Autodesk Inventor part; units mm, degrees
ref_plane "YZ Plane" through (0, 0, 0) normal (1, 0, 0) x (0, 1, 0)
ref_plane "XZ Plane" through (0, 0, 0) normal (0, 1, 0) x (-1, 0, 0)
ref_plane "XY Plane" through (0, 0, 0) normal (0, 0, 1) x (1, 0, 0)
sketch "Sketch1" plane through (0, 0, 0) normal (0, 0, 1) x (1, 0, 0)
  arc A0 (1.4, -1.4283) -> (-1.4, -1.4283) centre (0, 0) ccw
  line L0 (-1.4, -1.4283) -> (-1.4, -10)
  line L1 (-1.4, -10) -> (1.4, -10)
  line L2 (1.4, -10) -> (1.4, -1.4283)
  point P0 (0, -10)
  dimension "d0" = 4
  dimension "d1" = 2.8
  dimension "d2" = 12
extrude "Extrusion1" add sketch "Sketch1" along normal blind 0.3
fillet "Fillet1" radius 1.4 2 edges at (1.4, -10, 0.15) (-1.4, -10, 0.15)
sketch "Sketch2" plane through (0, 0, 0.3) normal (0, 0, 1) x (1, 0, 0)
  circle A0 centre (0, -3.9283) radius 0.9
  point P0 (1.4, -1.4283)
  dimension "d6" = 1.8
  dimension "d7" = 2.5
extrude "Extrusion2" cut sketch "Sketch2" against normal through all
properties material "Brass, Soft Yellow"
Geometry: final body of the model. Coordinates: model frame, mm. Round coordinates to 2 decimals unless told otherwise and drop trailing zeros. Order: outer loops, then holes, each group sorted by start corner. A loop starts at its lowest first (then second) coordinate and runs counter-clockwise, first axis right, second up. Notation, with made-up numbers: (-17.75, -32) -> (-0.75, -32) arc R34 cw to (-0.75, 7) -> close; hole circle Ø9 at (-13.75, -0.5). An arc over 180 degrees is marked (long way). Put each result on its own line as item: value. Start each with the question number.
Q1. Section D-D on y = -8.75. Return the cut outline in (x, z), and give its area (3 significant figures).
Q2. First-contact query: pin 1 (1 mm diameter, centred on x = 1.5, y = -3, fed in from -Z). Flat tip, straight axial feed; report the tip coordinate or a pass-through.
Q3. Section A-A on y = -3.5. Return the cut outline in (x, z), and give its area (3 significant figures).
Q4. Line query: probe 1 along X at (y, z) = (-6.5, 0.15); probe 2 along Y at (x, z) = (0.7, 0.15); probe 3 along X at (y, z) = (0.5, 0.1). Output: solid intervals per line, ascending.
Q5. Section B-B on x = -0.5. Return the cut outline in (y, z).
Ans:
1. outline: (-1.39, 0) -> (1.39, 0) -> (1.39, 0.3) -> (-1.39, 0.3) -> close
1. area: 0.835 mm2
2. pin 1: stops at z = 0
3. outline: (-1.4, 0) -> (-0.79, 0) -> (-0.79, 0.3) -> (-1.4, 0.3) -> close; (0.79, 0) -> (1.4, 0) -> (1.4, 0.3) -> (0.79, 0.3) -> close
3. area: 0.365 mm2
4. probe 1: x = -1.4 to 1.4
4. probe 2: y = -9.81 to -4.49, -3.36 to 1.87
4. probe 3: x = -1.94 to 1.94
5. outline: (-9.91, 0) -> (-4.68, 0) -> (-4.68, 0.3) -> (-9.91, 0.3) -> close; (-3.18, 0) -> (1.94, 0) -> (1.94, 0.3) -> (-3.18, 0.3) -> close
